Drawing for the job (mm, zero at the part's lowest x, y, z). A direction names the side the tool comes from. Round coordinates to 2 decimals unless told otherwise and drop trailing zeros. Write each loop counter-clockwise with the first axis right and the second up, starting at its lowest first coordinate (ties: lowest second). Pieces come first, ordered by that corner, then holes. Notation, with made-up numbers: (11, 2) - (34, 2) arc R9 ccw to (34, 14) - close; hole circle Ø3 at (22, -34.75). An arc over 180 degrees is marked (long way). Answer in a Markdown table with one row per item.
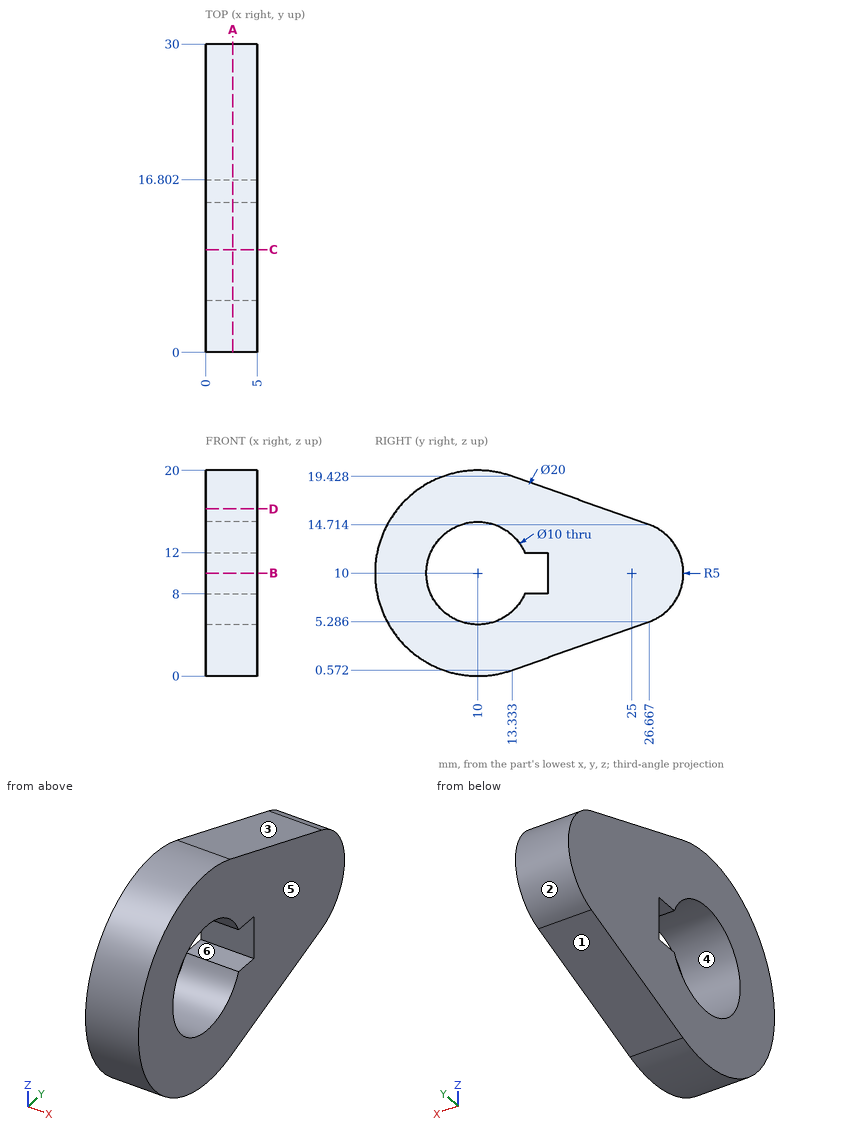
Q1. Saw through at C-C on y = 10. List the corners of the cut face in (x, z).
Computed:
| item | result |
|---|---|
| outline | (0, 0) - (5, 0) - (5, 5) - (0, 5) - close; (0, 15) - (5, 15) - (5, 20) - (0, 20) - close |
Q2. Saw through at A-A on x = 2.65. List the corners of the cut face in (y, z).
Computed:
| item | result |
|---|---|
| outline | (13.33, 0.57) - (26.67, 5.29) arc R5 ccw to (26.67, 14.71) - (13.33, 19.43) arc R10 ccw (long way) to start; hole (14.58, 8) - (16.8, 8) - (16.8, 12) - (14.58, 12) arc R5 ccw (long way) to start |
Q3. Saw through at B-B on z = 10. List the corners of the cut face in (x, y), then the cut area to 3 significant figures.
Computed:
| item | result |
|---|---|
| outline | (0, 0) - (5, 0) - (5, 5) - (0, 5) - close; (0, 16.8) - (5, 16.8) - (5, 30) - (0, 30) - close |
| area | 91.0 mm2 |
Q4. Drill centre lines: line 1 (Z direction, x = 3.3, y = 10); line 2 (Y direction, x = 1.3, z = 14.5); line 3 (Y direction, x = 2.85, z = 7.25) (1 decimal). Where is each one in solid material? Low to high.
Computed:
| item | result |
|---|---|
| line 1 | z = 0 to 5, 15 to 20 |
| line 2 | y = 1.07 to 7.82, 12.18 to 27.18 |
| line 3 | y = 0.4 to 5.8, 14.2 to 29.2 |
Q5. Pull direction Z, two halves, no side cores. Call the marked faces 1, 2, 3 and 4: released by +Z, released by -Z, zero draft, split by the parting line, or undercut.
Computed:
| item | result |
|---|---|
| face 1 | released by -Z |
| face 2 | split by the parting line |
| face 3 | released by +Z |
| face 4 | undercut |
Q6. 3-axis set-ups, long thin cutter, end or side, ignore diameter. For the marked faces 5 and 6: which of +Z, -Z, +X, -X, +Y, -Y reach the whole face in a straight line?
Computed:
| item | result |
|---|---|
| face 5 | +Z, -Z, +X, +Y, -Y |
| face 6 | +X, -X |
Q7. Flat gauge pins, fed straight in: pin 1 (2.5 mm diameter, centred on x = 3.5, y = 16, fed in from -Z); pin 2 (2 mm diameter, centred on x = 4, y = 25, fed in from -Z); pin 3 (1.8 mm diameter, centred on x = 2, y = 15.5, fed in from +Z). Where does each tip first touch, or does it go through?
Computed:
| item | result |
|---|---|
| pin 1 | stops at z = 1.07 |
| pin 2 | stops at z = 4.34 |
| pin 3 | stops at z = 18.98 |
Q8. Saw through at D-D on z = 16.25. List the corners of the cut face in (x, y).
Computed:
| item | result |
|---|---|
| outline | (0, 2.19) - (5, 2.19) - (5, 22.32) - (0, 22.32) - close |
